For this review, use the dimensioned drawing (mm, ordinates from the lowest corner) and the shaded views. A direction names the side the tool comes from. Give positions to 0.01 mm unless a question says otherwise; leave off trailing zeros. Order: outer loops, then holes, each group sorted by start corner. A loop starts at its lowest first (then second) coordinate and runs counter-clockwise, first axis right, second up. Notation, with made-up numbers: (-18.75, 74.5) - (2.25, 74.5) arc R7 ccw to (2.25, 84.5) - close; hole circle Ø4 at (38, -26). An arc over 180 degrees is marked (long way). One line per item, written item: value.
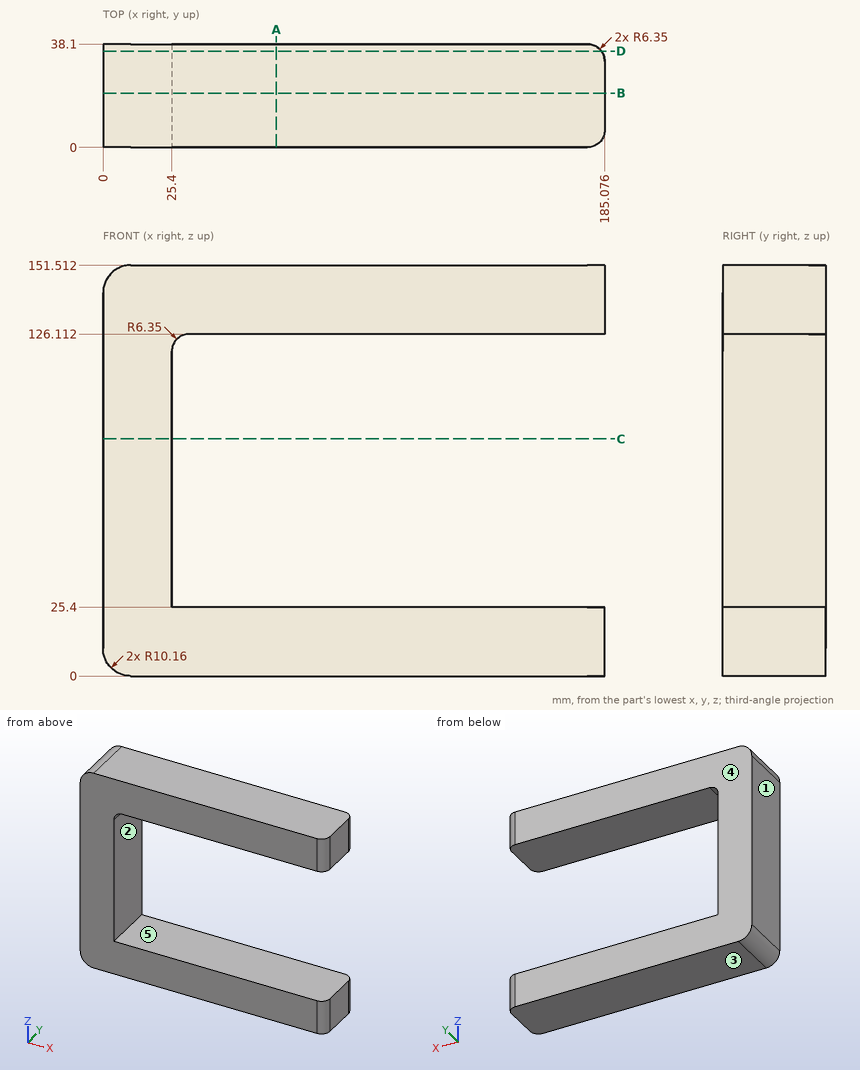
(1) Wall thickness on line 1 (Z direction, x = 165, y = 10); line 2 (X direction, y = 33, z = 110); line 3 (X direction, y = 3, z = 137): over which ranges is each line inside the solid? List them lowest first. Write a range as from..to.
Answers below:
line 1: z = 0..25.4, 126.11..151.51
line 2: x = 0..25.4
line 3: x = 0..184.12
(2) For P1, Ø12, axis at x = 58.5, z = 124, coming from the +Y side; P2, Ø11.5, axis at y = 23, z = 62, coming from the +X side, all flat-tipped, find the tip position at first contact; note any pin that passes through.
Answers below:
P1: stops at y = 38.1
P2: stops at x = 25.4
(3) Draft analysis for pull direction Z (two halves, no side actions). For the marked faces 1, 2 and 3, state which applies: pulls with the +Z half, pulls with the -Z half, needs draft (parallel to the pull), parting line crosses it, or undercut.
Answers below:
face 1: needs draft
face 2: undercut
face 3: pulls with the -Z half
(4) Take a section at D-D (y = 35.5). Write out the cut boundary in (x, z).
Answers below:
outline: (0, 10.16) arc R10.16 ccw to (10.16, 0) - (183.85, 0) - (183.85, 25.4) - (25.4, 25.4) - (25.4, 119.76) arc R6.35 cw to (31.75, 126.11) - (183.85, 126.11) - (183.85, 151.51) - (10.16, 151.51) arc R10.16 ccw to (0, 141.35) - close
(5) Take a section at B-B (y = 20). Write out the cut boundary in (x, z), then the cut area to 3 significant figures.
Answers below:
outline: (0, 10.16) arc R10.16 ccw to (10.16, 0) - (185.08, 0) - (185.08, 25.4) - (25.4, 25.4) - (25.4, 119.76) arc R6.35 cw to (31.75, 126.11) - (185.08, 126.11) - (185.08, 151.51) - (10.16, 151.51) arc R10.16 ccw to (0, 141.35) - close
area: 11,900 mm^2
(6) Take a section at C-C (z = 87.5). Write out the cut boundary in (x, y), then the cut area to 3 significant figures.
Answers below:
outline: (0, 0) - (25.4, 0) - (25.4, 38.1) - (0, 38.1) - close
area: 968 mm^2
(7) Take a section at A-A (x = 64). Write out the cut boundary in (y, z).
Answers below:
outline: (0, 0) - (38.1, 0) - (38.1, 25.4) - (0, 25.4) - close; (0, 126.11) - (38.1, 126.11) - (38.1, 151.51) - (0, 151.51) - close
(8) Machinability: for the marked faces 4 and 5, which of the approach directions +Z, -Z, +X, -X, +Y, -Y give a long, thin tool a straight path to every point of the face, cutting with its end or side? Answer none if there is none.
Answers below:
face 4: +Z, -Z, +X, -X, +Y
face 5: +X, +Y, -Y
